from build123d import *

# Parameters (mm, degrees)
SKETCH3_W               = 114.3
SKETCH3_H               = 38.1
BOSS_EXTRUDE1_DEPTH     = 3.81
BOSS_EXTRUDE2_START     = -19.05
BOSS_EXTRUDE2_OUTLINE_R = 13.5453125
BOSS_EXTRUDE2_DEPTH     = 38.1
FILLET1_R               = 2.032
SKETCH5_R               = 2.749999961
CUT_EXTRUDE4_DEPTH      = 12.7
SKETCH6_R               = 2.749999961
CUT_EXTRUDE5_DEPTH      = 7.62


# Read off the part's stored shape, not the designer's step: Boss-Extrude2
with BuildPart() as part:
    # Sketch3 → Boss-Extrude1 (new body)
    with BuildSketch(Plane(origin=(0, 0, 0), x_dir=(1, 0, 0), z_dir=(0, 1, 0))):
        Rectangle(SKETCH3_W, SKETCH3_H)
    extrude(amount=BOSS_EXTRUDE1_DEPTH)

    # Boss-Extrude2 outline → Boss-Extrude2 (add)
    # profile 1 of 2: a face of its own
    with BuildSketch(Plane.XY.offset(BOSS_EXTRUDE2_START)):
        with BuildLine():
            ThreePointArc((58.658787305, 0), (76.014099805, 17.3553125), (58.658787305, 34.710625))
            Line((58.658787305, 34.710625), (58.658787305, 30.900625))
            ThreePointArc((58.658787305, 30.900625), (69.035098676, 8.648553456), (45.319258538, 15.003193668))
            Line((45.319258538, 15.003193668), (41.567140999, 14.341594112))
            ThreePointArc((41.567140999, 14.341594112), (41.806974837, 13.2052175), (42.122274879, 12.087425946))
            ThreePointArc((42.122274879, 12.087425946), (41.198342199, 6.412778013), (36.071859255, 3.81))
            Line((36.071859255, 3.81), (57.15, 3.81))
            Line((57.15, 3.81), (57.15, 0))
            Line((57.15, 0), (58.658787305, 0))
        make_face()
    # profile 2 of 2: a face of its own
    with BuildSketch(Plane.XY.offset(BOSS_EXTRUDE2_START)):
        with BuildLine():
            Line((-58.658787305, 0), (-57.15, 0))
            Line((-57.15, 0), (-57.15, 3.81))
            Line((-57.15, 3.81), (-36.071859255, 3.81))
            ThreePointArc((-36.071859255, 3.81), (-41.198342199, 6.412778013), (-42.122274879, 12.087425946))
            ThreePointArc((-42.122274879, 12.087425946), (-49.981131055, 32.385454016), (-71.489167098, 29.042409074))
            ThreePointArc((-71.489167098, 29.042409074), (-76.865522705, 27.00523428), (-81.682836057, 30.143509735))
            Line((-81.682836057, 30.143509735), (-117.754695312, 92.621802688))
            ThreePointArc((-117.754695312, 92.621802688), (-118.063864905, 98.362856156), (-113.611441977, 102.000329294))
            ThreePointArc((-113.611441977, 102.000329294), (-112.485756074, 102.286167225), (-111.381708141, 102.646653335))
            Line((-111.381708141, 102.646653335), (-112.684804887, 106.22688222))
            ThreePointArc((-112.684804887, 106.22688222), (-130.046004812, 123.588082145), (-105.586989883, 125.727968673))
            Line((-105.586989883, 125.727968673), (-102.287433094, 127.632968673))
            ThreePointArc((-102.287433094, 127.632968673), (-125.99523086, 133.985453938), (-132.347716126, 110.277656173))
            Line((-132.347716126, 110.277656173), (-73.688928821, 8.67765625))
            ThreePointArc((-73.688928821, 8.67765625), (-67.336443555, 2.325170984), (-58.658787305, 0))
        make_face()
        with Locations((-58.658787305, 17.3553125)):
            Circle(BOSS_EXTRUDE2_OUTLINE_R, mode=Mode.SUBTRACT)
    extrude(amount=BOSS_EXTRUDE2_DEPTH)

    # Fillet1
    # the kernel refuses this fillet: 2.032 mm, written as the material it takes off along each edge
    with BuildSketch(Plane(origin=(58.658787305, 34.710625, -24.816396244), x_dir=(0.9977896842762429, -0.06645107938864002, 0), z_dir=(0, 0, 1))) as fillet1_piece_1:
        with BuildLine():
            CenterArc((2.171529904, -2.027508638), FILLET1_R, 86.189825964, 97.620348072)
            Line((0.144021266, -2.162537232), (0, 0))
            ThreePointArc((0, 0), (1.153279249, 0.03836072), (2.306558498, 0))
        make_face()
    extrude(amount=49.632792488, mode=Mode.SUBTRACT)
    with BuildSketch(Plane(origin=(58.658787305, 30.900625, -23.797245223), x_dir=(0, 1, 0), z_dir=(0, 0, 1)), Plane(origin=(-112.684804887, 106.22688222, -23.797245223), x_dir=(0.342020143325642, -0.9396926207859182, 0), z_dir=(0, 0, 1))) as fillet1_piece_2:
        with BuildLine():
            CenterArc((1.898898089, -2.032), FILLET1_R, 90, 82.504627273)
            ThreePointArc((-0.115739283, -1.766933481), (-0.028965791, -0.885360027), (0, 0))
            Line((0, 0), (1.898898089, 0))
        make_face()
    extrude(amount=47.594490446, mode=Mode.SUBTRACT)
    with BuildSketch(Plane(origin=(45.319258538, 15.003193668, -23.797245222), x_dir=(0.23764666879808158, -0.9713516669101747, 0), z_dir=(0, 0, 1))) as fillet1_piece_3:
        with BuildLine():
            CenterArc((1.903537334, -2.027654697), FILLET1_R, 93.747686362, 82.50462726)
            Line((-0.124117363, -1.894837416), (0, 0))
            ThreePointArc((0, 0), (0.885360027, -0.028965791), (1.770720053, 0))
        make_face()
    extrude(amount=47.594490443, mode=Mode.SUBTRACT)
    with BuildSketch(Plane(origin=(41.567140999, 14.341594112, -24.816396246), x_dir=(0.984807753053284, 0.17364817743397684, 0), z_dir=(0, 0, 1))) as fillet1_piece_4:
        with BuildLine():
            CenterArc((2.167327711, -2.032), FILLET1_R, 90, 97.620348093)
            ThreePointArc((0.153273303, -2.301460276), (0.038360721, -1.153279249), (0, 0))
            Line((0, 0), (2.167327711, 0))
        make_face()
    extrude(amount=49.632792491, mode=Mode.SUBTRACT)
    with BuildSketch(Plane(origin=(-102.287433094, 127.632968673, -24.816396244), x_dir=(-0.8660254038225857, -0.4999999999339274, 0), z_dir=(0, 0, 1))) as fillet1_piece_5:
        with BuildLine():
            CenterArc((2.167327711, -2.032), FILLET1_R, 90, 97.62034808)
            ThreePointArc((0.153273302, -2.301460275), (0.03836072, -1.153279249), (0, 0))
            Line((0, 0), (2.167327711, 0))
        make_face()
    extrude(amount=49.632792489, mode=Mode.SUBTRACT)
    with BuildSketch(Plane(origin=(-105.586989883, 125.727968673, -23.797245222), x_dir=(-0.5555366573888737, 0.8314920458412077, 0), z_dir=(0, 0, 1))) as fillet1_piece_6:
        with BuildLine():
            CenterArc((1.903537334, -2.027654697), FILLET1_R, 93.747686363, 82.504627266)
            Line((-0.124117363, -1.894837416), (0, 0))
            ThreePointArc((0, 0), (0.885360027, -0.028965791), (1.770720053, 0))
        make_face()
    extrude(amount=47.594490445, mode=Mode.SUBTRACT)
    with BuildSketch(Plane(origin=(-111.381708141, 102.646653335, -24.816396244), x_dir=(-0.960343211064482, -0.2788205820278691, 0), z_dir=(0, 0, 1))) as fillet1_piece_7:
        with BuildLine():
            CenterArc((2.171529904, -2.027508638), FILLET1_R, 86.189825951, 97.620348077)
            Line((0.144021265, -2.162537231), (0, 0))
            ThreePointArc((0, 0), (1.153279249, 0.03836072), (2.306558498, 0))
        make_face()
    extrude(amount=49.632792488, mode=Mode.SUBTRACT)

    # Sketch5 → Cut-Extrude4 (cut)
    with BuildSketch(Plane(origin=(0, 3.81, 0), x_dir=(1, 0, 0), z_dir=(0, 1, 0))):
        with Locations(Location((-17.78, 0, 0), (0, 0, 270))):
            Circle(SKETCH5_R)
        with Locations(Location((3.81, 0, 0), (0, 0, 270))):
            Circle(SKETCH5_R)
    extrude(amount=-CUT_EXTRUDE4_DEPTH, mode=Mode.SUBTRACT)

    # Sketch6 → Cut-Extrude5 (cut)
    with BuildSketch(Plane(origin=(-48.209604448, -27.833828106, 0), x_dir=(0, 0, -1), z_dir=(0.8660254037844433, 0.4999999999999923, 0))):
        with Locations(Location((-10.795, 85.238322473, 0), (0, 0, 90))):
            Circle(SKETCH6_R)
        with Locations(Location((10.795, 85.238322473, 0), (0, 0, 90))):
            Circle(SKETCH6_R)
    extrude(amount=-CUT_EXTRUDE5_DEPTH, mode=Mode.SUBTRACT)


solid = part.part
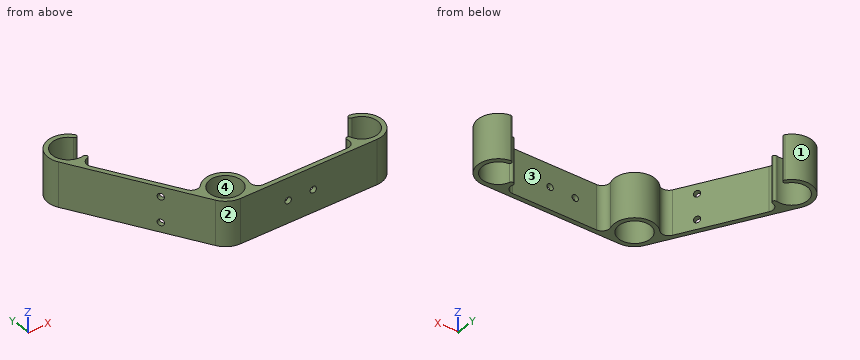
Source: CAD feature listing. Evaluate the final solid. Frame: model axes, mm. Face numbers are marked on the shaded views. Give positions to 0.01 mm unless a question says otherwise; leave off trailing zeros. Order: outer loops, then holes, each group sorted by start corner. A loop starts at its lowest first (then second) coordinate and runs counter-clockwise, first axis right, second up. Notation, with made-up numbers: (-5, 73) -> (35, 73) arc R13 cw to (35, 88) -> close; hole circle Ø5 at (-29, -16). An arc over 180 degrees is marked (long way). Write item = value, one per line.
Q1. Cut plane D-D, the plane y = 116.5. Output: boundary loops of the cut face in (x, z), and give its area (3 significant figures).
Data:
outline = (-134.5, -19.05) -> (-130.64, -19.05) -> (-130.64, 19.05) -> (-134.5, 19.05) -> close
area = 147 mm^2
Q2. Pin query (flat end, axial travel): pin 1 (6 mm diameter, centred on y = 121.5, z = -5.5, fed in from +X); pin 2 (2 mm diameter, centred on y = 34.5, z = -14, fed in from -X); pin 3 (4 mm diameter, centred on y = 62.5, z = -6.5, fed in from +X). Return the tip coordinate at first contact, or that it passes through.
Data:
pin_1 = -129.68
pin_2 = -89.17
pin_3 = -99.21
Q3. Material intervals for line 1 (X direction, y = 19.5, z = -12.5); line 2 (X direction, y = 29.5, z = -10.5); line 3 (Y direction, x = 19.5, z = -5), sorted ascending. Write a range as from..to.
Data:
line_1 = -79.94..-72.03, -45.28..-41.44, 72.03..75.88
line_2 = -85.71..-81.26, -71.06..-64.66, -52.66..-46.26, 64.66..71.06
line_3 = 0..3.81
Q4. Pull-direction query (Y, two-part tool) for the marked faces 1, 2, 3 and 4; classes: released by +Y, released by -Y, zero draft, split by the parting line, or undercut.
Data:
face_1 = split by the parting line
face_2 = released by -Y
face_3 = released by +Y
face_4 = undercut
Q5. Cut plane B-B, the plane z = 0. State how many separate pieces and enclosed holes the cut face has, and give its area (3 significant figures).
Data:
separate_pieces = 3
enclosed_holes = 1
area = 1,740 mm^2
Q6. Cut plane C-C, the plane x = 22. Output: boundary loops of the cut face in (y, z).
Data:
outline = (0, -19.05) -> (3.81, -19.05) -> (3.81, 19.05) -> (0, 19.05) -> close
Q7. Cut plane A-A, the plane x = -17.78. Output: boundary loops of the cut face in (y, z).
Data:
outline = (0, -19.05) -> (3.81, -19.05) -> (3.81, -2.75) -> (0, -2.75) -> close; (0, 2.75) -> (3.81, 2.75) -> (3.81, 19.05) -> (0, 19.05) -> close
